Autodesk Inventor part; units mm, degrees
ref_plane "YZ Plane" through (0, 0, 0) normal (1, 0, 0) x (0, 1, 0)
ref_plane "XZ Plane" through (0, 0, 0) normal (0, 1, 0) x (-1, 0, 0)
ref_plane "XY Plane" through (0, 0, 0) normal (0, 0, 1) x (1, 0, 0)
sketch "Sketch1" plane through (0, 0, 0) normal (0, 0, 1) x (1, 0, 0)
  line L0 (-3.5, 0) -> (-3.5, -20)
  line L1 (-3.5, -20) -> (0, -20)
  line L2 (-16.2, -20) -> (-16.2, 4)
  line L3 (-16.2, -20) -> (-12.7, -20)
  line L4 (-12.7, 0) -> (-12.7, -20)
  line L5 (0, 4) -> (-16.2, 4)
  line L6 (-16.2, 4) -> (-16.2, -15.5962)
  line L7 (-16.2, -15.5962) -> (0, -15.5962)
  line L8 (0, -15.5962) -> (0, 4)
  line L9 (0, -20) -> (0, 4)
  line L10 (-16.2, 4) -> (0, 4)
  line L11 (-12.7, 0) -> (-3.5, 0)
  point P0 (0, 0)
  point P1 (-12.7, -15.5962)
  point P2 (-3.5, -15.5962)
extrude "Extrusion1" add sketch "Sketch1" along normal blind 2 contours L11 L4 L7 L2 L5 L8 L0 | L0 L7 L4 L11 | L4 L3 L2 L7
sketch "Sketch2" plane through (0, 0, 2) normal (0, 0, 1) x (1, 0, 0)
  line L0 (0, -15.5962) -> (0, 4)
  line L1 (0, 4) -> (-16.2, 4)
  line L2 (-16.2, 4) -> (-16.2, -20)
  line L3 (-12.7, -15.5962) -> (0, -15.5962)
  circle A0 centre (-8.1, -11.6475) radius 1
  line L4 (-12.7, -20) -> (-12.7, -15.5962)
  line L5 (-16.2, -20) -> (-12.7, -20)
  point P0 (0, 0)
  dimension "d2" = 2
extrude "Extrusion2" add sketch "Sketch2" against normal blind 10 contours A0
chamfer "Chamfer1" distance 1 angle 45 1 edges at (-9.1, -11.6475, -8)
pattern_linear "Rectangular Pattern1" [suppressed]
properties part number "30_XY_Sample_lightsheetarm_sample_lid"
CAD build for the part. Positions are in the model's coordinates, mm. A direction names the side the tool comes from. Round coordinates to 2 decimals unless told otherwise and drop trailing zeros. Write each loop counter-clockwise with the first axis right and the second up, starting at its lowest first coordinate (ties: lowest second). Pieces come first, ordered by that corner, then holes. Notation, with made-up numbers: (-30, -39.75) - (24, -39.75) arc R22 ccw to (24, -21.75) - close; hole circle Ø11 at (-11, -29.75). An arc over 180 degrees is marked (long way). Write item = value, one per line. Start each with the question number.
Q1. Which spindle directions (+Z, -Z, +X, -X, +Y, -Y) get a long thin tool onto all of the face, cutting with end or side? Do faces 1 (the cylindrical face through (-8.89, -12.26, -3.45)), 2 (the flat face through (-6, -15.596, 1)), 3 (the flat face through (-8, -5, 2)). Say none if no direction does.
Q2. Probe L1, parallel to Z at x = -10, y = -10.5; L2, parallel to Y at x = -6.25, z = 0.5. List the from-to ranges inside material, lowest first. Write a range as from..to.
Q3. Band-saw the part on A-A (x = -13.5). Give the cut face in (y, z).
Q4. Drop flat-ended pins along their axis: pin 1 (4 mm diameter, centred on x = -8, z = -0.5, fed in from -Y); pin 2 (1.6 mm diameter, centred on y = -17, z = 1, fed in from +X); pin 3 (8 mm diameter, centred on x = -11, y = -7.5, fed in from -Z); pin 4 (1.5 mm diameter, centred on y = -13.5, z = -6, fed in from +X). Give the stop position or say it passes through.
Q5. Band-saw the part on C-C (z = -1). Give the cut face in (x, y), then the cut area to 3 significant figures.
Q6. Band-saw the part on B-B (y = -16). Give the cut face in (x, z), then the cut area to 3 significant figures.
Answers below:
q1.face_1 = -Z
q1.face_2 = +Z, -Z, +X, -Y
q1.face_3 = +Z, +X, -X, +Y, -Y
q2.L1 = 0..2
q2.L2 = -15.6..4
q3.outline = (-20, 0) - (4, 0) - (4, 2) - (-20, 2) - close
q4.pin_1 = -15.6
q4.pin_2 = -12.7
q4.pin_3 = 0
q4.pin_4 = through
q5.outline = circle Ø2 at (-8.1, -11.65)
q5.area = 3.14 mm2
q6.outline = (-16.2, 0) - (-12.7, 0) - (-12.7, 2) - (-16.2, 2) - close
q6.area = 7.00 mm2
